```python
from build123d import *

# Parameters (mm, degrees)
SKETCH1_W                                    = 131.06
SKETCH1_H                                    = 88.78
BOSS_EXTRUDE1_DEPTH                          = 5
SKETCH2_W                                    = 131.06
SKETCH2_H                                    = 88.78
SKETCH2_W_2                                  = 125.06
SKETCH2_H_2                                  = 82.78
BOSS_EXTRUDE2_DEPTH                          = 5
CHAMFER1_SIZE                                = 2
CUT_EXTRUDE1_DEPTH                           = 80.307332574
BOSS_EXTRUDE3_START                          = -44.39
BOSS_EXTRUDE3_DEPTH                          = 88.78
BOSS_EXTRUDE4_DEPTH                          = 5
CBORE_FOR_M4_HEX_HEAD_CAP_SCREW1_D           = 4.5
CBORE_FOR_M4_HEX_HEAD_CAP_SCREW1_CBORE_D     = 11.083
CBORE_FOR_M4_HEX_HEAD_CAP_SCREW1_CBORE_DEPTH = 2.8


with BuildPart() as part:
    # Sketch1 → Boss-Extrude1 (new body)
    with BuildSketch(Plane(origin=(0, 0, 0), x_dir=(1, 0, 0), z_dir=(0, 1, 0))):
        Rectangle(SKETCH1_W, SKETCH1_H)
    extrude(amount=BOSS_EXTRUDE1_DEPTH)

    # Sketch2 → Boss-Extrude2 (add)
    with BuildSketch(Plane(origin=(0, 5, 0), x_dir=(1, 0, 0), z_dir=(0, 1, 0))):
        Rectangle(SKETCH2_W, SKETCH2_H)
        Rectangle(SKETCH2_W_2, SKETCH2_H_2, mode=Mode.SUBTRACT)
    extrude(amount=BOSS_EXTRUDE2_DEPTH)

    # Chamfer1
    chamfer1_edges = [part.edges().sort_by_distance(p)[0] for p in [
        (62.53, 10, 0),
        (0, 10, -41.39),
        (-62.53, 10, 0),
        (0, 10, 41.39),
    ]]
    chamfer(chamfer1_edges, length=CHAMFER1_SIZE)

    # Sketch3 → Cut-Extrude1 (cut, through all)
    with BuildSketch(Plane(origin=(0, 5, 0), x_dir=(1, 0, 0), z_dir=(0, 1, 0))):
        Polygon((-65.53, 32.39), (-65.53, -32.39), (-53.53, -32.39), (-53.53, -44.39), (53.53, -44.39), (53.53, -32.39), (65.53, -32.39), (65.53, 32.39), (53.53, 32.39), (53.53, 44.39), (-53.53, 44.39), (-53.53, 32.39), align=None)
    extrude(amount=CUT_EXTRUDE1_DEPTH, mode=Mode.SUBTRACT)

    # Sketch4 → Boss-Extrude3 (add)
    with BuildSketch(Plane.XY.offset(BOSS_EXTRUDE3_START)):
        Polygon((65.53, 0), (65.53, -50), (55.53, -50), (55.53, -20), (25.33, -20), (25.33, -30), (15.33, -30), (15.33, 0), align=None)
    extrude(amount=BOSS_EXTRUDE3_DEPTH)

    # Sketch5 → Boss-Extrude4 (add)
    with BuildSketch(Plane.XY.offset(44.39)):
        Polygon((-65.53, 0), (15.33, -30), (15.33, 0), align=None)
    boss_extrude4 = extrude(amount=-BOSS_EXTRUDE4_DEPTH)

    # Mirror1: Boss-Extrude4 across plane
    add(boss_extrude4.mirror(Plane.XY))

    # CBORE for M4 Hex Head Cap Screw1 (through all)
    with Locations(Plane(origin=(65.53, 0, 0), x_dir=(0, 0, -1), z_dir=(1, 0, 0))):
        with Locations((-24.39, -35), (24.39, -35)):
            CounterBoreHole(CBORE_FOR_M4_HEX_HEAD_CAP_SCREW1_D / 2, CBORE_FOR_M4_HEX_HEAD_CAP_SCREW1_CBORE_D / 2, CBORE_FOR_M4_HEX_HEAD_CAP_SCREW1_CBORE_DEPTH)


solid = part.part
```
Geometry: final body of the model. Coordinates: model frame, mm. A direction names the side the tool comes from. Coordinates: 2 decimals unless noted, no trailing zeros. Order: outer loops, then holes, each group sorted by start corner. A loop starts at its lowest first (then second) coordinate and runs counter-clockwise, first axis right, second up. Notation, with made-up numbers: M 30.5,49 L 41.5,49 A32 ccw 41.5,84 Z; hole C 65,26.5 d1. An arc over 180 degrees is marked long. Answer in a Markdown table with one row per item. Add a question column.
Q1. Mould query, pull axis Z, two halves, no side actions, for faces 5 (the flat face through (53.53, 7, -43)), 6 (the flat face through (-64, 7, -32.39)). Classes: released by +Z, released by -Z, zero draft, split by the parting line, or undercut.
Q2. Reachability of faces 1 (the flat face through (53.53, 7, 43)), 2 (the flat face through (-58, 6, -41.39)), 3 (the flat face through (-8, -8, 39.39)), 4 (the flat face through (25.33, -25, -1)) from +Z, -Z, +X, -X, +Y, -Y: full face, straight path, thin tool, end or side. Return the list, or none.
Q3. Contact query for flat-ended pins moving along their axis: P1, Ø8, axis at y = -32.5, z = 6, coming from the -X side; P2, Ø5, axis at x = -52.5, z = 2.5, coming from the +Y side; P3, Ø4, axis at x = 34, z = -23, coming from the -Y side. Output: stop coordinate, or through.
Q4. Line query: L1, parallel to X at y = -25, z = -3.5; L2, parallel to Y at x = 64, z = 24; L3, parallel to Z at x = -36, y = -1. Output: solid intervals per line, ascending.
Q5. Section query B-B on z = -24.39. Return the cut outline in (x, y), and give its area (3 significant figures).
Q6. Section query C-C on x = 3.5. Return the cut outline in (y, z), and give its area (3 significant figures).
Q7. Section query A-A on y = -35. Return the cut outline in (x, z).
Q8. Section query D-D on z = 38. Return the cut outline in (x, y).
Completed:
| question | item | result |
|---|---|---|
| 1 | face 5 | zero draft |
| 1 | face 6 | undercut |
| 2 | face 1 | +Z, -Z, +Y |
| 2 | face 2 | +Y |
| 2 | face 3 | -X, -Y |
| 2 | face 4 | +Z, -Z, -Y |
| 3 | P1 | stops at x = 15.33 |
| 3 | P2 | stops at y = 5 |
| 3 | P3 | stops at y = -20 |
| 4 | L1 | x = 15.33 to 25.33, 55.53 to 65.53 |
| 4 | L2 | y = -50 to -40.53, -29.47 to 5 |
| 4 | L3 | z = -44.39 to -39.39, 39.39 to 44.39 |
| 5 | outline | M -65.53,0 L 15.33,0 L 15.33,-30 L 25.33,-30 L 25.33,-20 L 55.53,-20 L 55.53,-32.75 L 62.73,-32.75 L 62.73,-29.46 L 65.53,-29.46 L 65.53,5 L -65.53,5 Z; M 55.53,-50 L 65.53,-50 L 65.53,-40.54 L 62.73,-40.54 L 62.73,-37.25 L 55.53,-37.25 Z |
| 5 | area | 2,000 mm2 |
| 6 | outline | M -25.61,-44.39 L 5,-44.39 L 5,44.39 L -25.61,44.39 L -25.61,39.39 L 0,39.39 L 0,-39.39 L -25.61,-39.39 Z |
| 6 | area | 700 mm2 |
| 7 | outline | M 55.53,-44.39 L 65.53,-44.39 L 65.53,-29.93 L 62.73,-29.93 L 62.73,-26.64 L 55.53,-26.64 Z; M 55.53,-22.14 L 62.73,-22.14 L 62.73,-18.85 L 65.53,-18.85 L 65.53,18.85 L 62.73,18.85 L 62.73,22.14 L 55.53,22.14 Z; M 55.53,26.64 L 62.73,26.64 L 62.73,29.93 L 65.53,29.93 L 65.53,44.39 L 55.53,44.39 Z |
| 8 | outline | M -65.53,0 L 15.33,0 L 15.33,-30 L 25.33,-30 L 25.33,-20 L 55.53,-20 L 55.53,-50 L 65.53,-50 L 65.53,10 L 64.53,10 L 62.53,8 L 62.53,5 L -62.53,5 L -62.53,8 L -64.53,10 L -65.53,10 Z |
